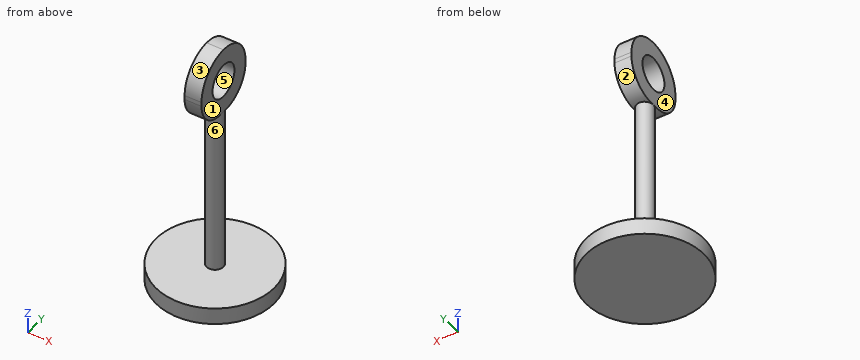
Autodesk Inventor part; units mm, degrees
ref_plane "YZ Plane" through (0, 0, 0) normal (1, 0, 0) x (0, 1, 0)
ref_plane "XZ Plane" through (0, 0, 0) normal (0, 1, 0) x (-1, 0, 0)
ref_plane "XY Plane" through (0, 0, 0) normal (0, 0, 1) x (1, 0, 0)
sketch "Skizze1" plane through (0, 0, 0) normal (0, 0, 1) x (1, 0, 0)
  circle A0 centre (0, 0) radius 3.5
  dimension "d0" = 7
extrude "Extrusion1" add sketch "Skizze1" along normal blind 1
sketch "Skizze2" plane through (0, 0, 1) normal (0, 0, 1) x (1, 0, 0)
  circle A0 centre (0, 0) radius 0.5
  dimension "d3" = 1
extrude "Extrusion2" add sketch "Skizze2" along normal blind 14
sketch "Skizze4" plane through (0, 0, 15) normal (0, 0, 1) x (1, 0, 0)
  line L0 (-0.5, -2) -> (0.5, -2)
  line L1 (0.5, -2) -> (0.5, 2)
  line L2 (0.5, 2) -> (-0.5, 2)
  line L3 (-0.5, 2) -> (-0.5, -2)
  circle A0 centre (0, 0) radius 0.5
  dimension "d25" = 1
  dimension "d26" = 4
  dimension "d27" = 2
extrude "Extrusion4" add sketch "Skizze4" against normal blind 4 contours L3 A0 L1 L0 | L3 L2 L1 A0
sketch "Skizze6" plane through (-0.5, -2, 15) normal (-1, 0, 0) x (0, 0, 1)
  circle A0 centre (-2, 2) radius 1
  line L0 (0, 4) -> (-4, 4)
  line L1 (0, 4) -> (0, 0)
  point P0 (-15, 2)
  dimension "d31" = 2
  dimension "d32" = 2
  dimension "d33" = 2
extrude "Extrusion5" cut sketch "Skizze6" against normal blind 1
sketch "Skizze10" plane through (-0.5, -2, 15) normal (-1, 0, 0) x (0, 0, 1)
  point P0 (-15, 2)
fillet "Rundung9" radius 2 1 edges at (0, 2, 15)
fillet "Rundung10" radius 2 1 edges at (0, -2, 15)
fillet "Rundung11" radius 1.75 1 edges at (0, -2, 11)
fillet "Rundung12" radius 1.75 1 edges at (0, 2, 11)
properties part number "Pneumatickolben_Kolbenkreis"
Check sheet for the modelled part. Datum: model origin and axes. Units: mm. Face numbers are marked on the shaded views. A direction names the side the tool comes from. Round coordinates to 2 decimals unless told otherwise and drop trailing zeros. Loops run counter-clockwise (first coordinate to the right, second up) from the corner with the lowest first, then second, coordinate; pieces in that order, holes last.
1. Sectioned sample at C-C on z = 13.75. Record the boundary of the cut face in (x, y).
2. Sectioned sample at B-B on y = 1.5. Record the boundary of the cut face in (x, z).
3. Sectioned sample at D-D on z = 2.25. Record the boundary of the cut face in (x, y), and give its area (3 significant figures).
4. Gauge pin test, flat ends, axial feed: pin 1 Ø3 at (y, z) = (0, 13) entering from +X; pin 2 Ø3 at (x, y) = (1.5, -0.5) entering from -Z; pin 3 Ø3 at (y, z) = (0, 13.5) entering from -X. Record the tip position at first contact, or that the pin passes through.
5. Scan lines: probe 1 along Y at (x, z) = (0.1, 13); probe 2 along Z at (x, y) = (0.75, -0.25); probe 3 along X at (y, z) = (-1.25, 12.75). Record each from-to range of solid material in increasing order.
6. Set-up check for the marked faces 4, 5 and 6: record each of +Z, -Z, +X, -X, +Y, -Y from which the full face is reachable in a straight line by a thin tool's end or side.
7. Mould release check, pull along Z, two halves, no side actions. Record for the marked faces 1, 2 and 3: released by +Z, released by -Z, zero draft, split by the parting line, or undercut.
Recorded:
1. outline: (-0.5, -1.85) - (0.5, -1.85) - (0.5, -0.66) - (-0.5, -0.66) - close; (-0.5, 0.66) - (0.5, 0.66) - (0.5, 1.85) - (-0.5, 1.85) - close
2. outline: (-3.16, 0) - (3.16, 0) - (3.16, 1) - (-3.16, 1) - close; (-0.5, 11.53) - (0.5, 11.53) - (0.5, 14.32) - (-0.5, 14.32) - close
3. outline: circle Ø1 at (0, 0)
3. area: 0.785 mm2
4. pin 1: stops at x = 0.5
4. pin 2: stops at z = 0
4. pin 3: stops at x = -0.5
5. probe 1: y = -2 to -1, 1 to 2
5. probe 2: z = 0 to 1
5. probe 3: x = -0.5 to 0.5
6. face 4: +Z, -X, +Y, -Y
6. face 5: +X, -X
6. face 6: none
7. face 1: zero draft
7. face 2: undercut
7. face 3: released by +Z
